CAD build for the part. Positions are in the model's coordinates, mm. Face numbers are marked on the shaded views. A direction names the side the tool comes from. Give positions to 0.01 mm unless a question says otherwise; leave off trailing zeros. Write each loop counter-clockwise with the first axis right and the second up, starting at its lowest first coordinate (ties: lowest second). Pieces come first, ordered by that corner, then holes. Notation, with made-up numbers: (63, 74) -> (118, 74) arc R24 cw to (118, 112) -> close; hole circle Ø4 at (1, -4). An arc over 180 degrees is marked (long way). Answer in a Markdown table with one row per item. Add a question column.
```python
from build123d import *

# Parameters (mm, degrees)
SKETCH1_R           = 1.8
SKETCH1_R_2         = 3.15
SKETCH1_R_3         = 8.05
SKETCH1_R_4         = 2.3
SKETCH1_R_5         = 19.05
SKETCH1_R_6         = 7.8
SKETCH1_R_7         = 1.3
SKETCH1_R_8         = 3.45
SKETCH1_W           = 98.2
SKETCH1_H           = 40.9
BOSS_EXTRUDE1_DEPTH = 3.2
BOSS_EXTRUDE2_START = 30
BOSS_EXTRUDE2_DEPTH = 30
FILLET1_R           = 4.8
SKETCH20_R          = 2.3
CUT_EXTRUDE8_DEPTH  = 10
SKETCH6_R           = 5
SKETCH6_R_2         = 2.3
BOSS_EXTRUDE3_DEPTH = 50
SKETCH12_W          = 192.98
SKETCH12_H          = 3.2
BOSS_EXTRUDE7_DEPTH = 15
SKETCH8_R           = 2.3
CUT_EXTRUDE2_DEPTH  = 10
SKETCH19_W          = 14
SKETCH19_H          = 60
CUT_EXTRUDE7_DEPTH  = 10
BOSS_EXTRUDE8_START = -30
SKETCH21_W          = 3.6
SKETCH21_H          = 22.135238484
SKETCH21_W_2        = 34.225238484
SKETCH21_H_2        = 3.6
BOSS_EXTRUDE8_DEPTH = 30
FILLET5_R           = 3
FILLET6_R           = 8


with BuildPart() as part:
    # Sketch1 → Boss-Extrude1 (new body)
    with BuildSketch(Plane(origin=(0, 0, 0), x_dir=(0, 0, -1), z_dir=(1, 0, 0))):
        with BuildLine():
            Line((-52.79, 54.2), (52.79, 54.2))
            ThreePointArc((52.79, 54.2), (91.185898218, 38.295898218), (107.09, -0.1))
            Line((107.09, -0.1), (107.09, -120.8))
            Line((107.09, -120.8), (-107.09, -120.8))
            Line((-107.09, -120.8), (-107.09, -0.1))
            ThreePointArc((-107.09, -0.1), (-91.185898218, 38.295898218), (-52.79, 54.2))
        make_face()
        with Locations((46.5, 27.4)):
            Circle(SKETCH1_R, mode=Mode.SUBTRACT)
        with Locations((-46.5, -27.6)):
            Circle(SKETCH1_R, mode=Mode.SUBTRACT)
        with Locations((-46.5, 27.4)):
            Circle(SKETCH1_R, mode=Mode.SUBTRACT)
        with Locations((46.5, -27.6)):
            Circle(SKETCH1_R, mode=Mode.SUBTRACT)
        with Locations((57.25, -0.1)):
            Circle(SKETCH1_R_2, mode=Mode.SUBTRACT)
        with Locations((68.55, -0.1)):
            Circle(SKETCH1_R_2, mode=Mode.SUBTRACT)
        with Locations((79.85, -0.1)):
            Circle(SKETCH1_R_2, mode=Mode.SUBTRACT)
        with Locations((91.15, -0.1)):
            Circle(SKETCH1_R_2, mode=Mode.SUBTRACT)
        with Locations((71.533650814, -45.1)):
            Circle(SKETCH1_R_3, mode=Mode.SUBTRACT)
        with Locations((87.09, -60.656349186)):
            Circle(SKETCH1_R_3, mode=Mode.SUBTRACT)
        with Locations((71.533650814, -76.212698372)):
            Circle(SKETCH1_R_3, mode=Mode.SUBTRACT)
        with Locations((55.977301628, -91.769047558)):
            Circle(SKETCH1_R_3, mode=Mode.SUBTRACT)
        with Locations((40.420952442, -107.325396744)):
            Circle(SKETCH1_R_3, mode=Mode.SUBTRACT)
        with Locations((55.977301628, -60.656349186)):
            Circle(SKETCH1_R_3, mode=Mode.SUBTRACT)
        with Locations((40.420952442, -76.212698372)):
            Circle(SKETCH1_R_3, mode=Mode.SUBTRACT)
        with Locations((24.864603256, -91.769047558)):
            Circle(SKETCH1_R_3, mode=Mode.SUBTRACT)
        with Locations((-87.45, -106.35)):
            Circle(SKETCH1_R_4, mode=Mode.SUBTRACT)
        with Locations((-52.45, -106.35)):
            Circle(SKETCH1_R_4, mode=Mode.SUBTRACT)
        with Locations((-52.45, -64.55)):
            Circle(SKETCH1_R_4, mode=Mode.SUBTRACT)
        with Locations((-87.45, -64.55)):
            Circle(SKETCH1_R_4, mode=Mode.SUBTRACT)
        with Locations((-69.1, -85.45)):
            Circle(SKETCH1_R_5, mode=Mode.SUBTRACT)
        with Locations((-81.9, -25.1)):
            Circle(SKETCH1_R_6, mode=Mode.SUBTRACT)
        with Locations((46.42, 37.2)):
            Circle(SKETCH1_R, mode=Mode.SUBTRACT)
        with Locations((0, 37.2)):
            Circle(SKETCH1_R, mode=Mode.SUBTRACT)
        with Locations((23.21, 34.55)):
            Circle(SKETCH1_R, mode=Mode.SUBTRACT)
        with Locations((23.21, -35.45)):
            Circle(SKETCH1_R, mode=Mode.SUBTRACT)
        with Locations((-29.2, -38.8)):
            Circle(SKETCH1_R_7, mode=Mode.SUBTRACT)
        with Locations((-13, -38.8)):
            Circle(SKETCH1_R_7, mode=Mode.SUBTRACT)
        with Locations((-13, -114.8)):
            Circle(SKETCH1_R_7, mode=Mode.SUBTRACT)
        with Locations((-29.2, -114.8)):
            Circle(SKETCH1_R_7, mode=Mode.SUBTRACT)
        with Locations((91.15, -12.7)):
            Circle(SKETCH1_R_8, mode=Mode.SUBTRACT)
        with Locations((79.85, -12.7)):
            Circle(SKETCH1_R_8, mode=Mode.SUBTRACT)
        with Locations((68.55, -12.7)):
            Circle(SKETCH1_R_8, mode=Mode.SUBTRACT)
        with Locations((57.25, -12.7)):
            Circle(SKETCH1_R_8, mode=Mode.SUBTRACT)
        Rectangle(SKETCH1_W, SKETCH1_H, mode=Mode.SUBTRACT)
    extrude(amount=BOSS_EXTRUDE1_DEPTH)

    # Sketch3 → Boss-Extrude2 (add)
    with BuildSketch(Plane.ZY.offset(BOSS_EXTRUDE2_START)):
        with BuildLine():
            Line((-107.09, -0.1), (-107.09, -120.8))
            Line((-107.09, -120.8), (107.09, -120.8))
            Line((107.09, -120.8), (107.09, -0.1))
            ThreePointArc((107.09, -0.1), (91.185898218, 38.295898218), (52.79, 54.2))
            Line((52.79, 54.2), (-52.79, 54.2))
            ThreePointArc((-52.79, 54.2), (-91.185898218, 38.295898218), (-107.09, -0.1))
        make_face()
        with BuildLine():
            Line((-103.89, -0.1), (-103.89, -117.6))
            Line((-103.89, -117.6), (103.89, -117.6))
            Line((103.89, -117.6), (103.89, -0.1))
            ThreePointArc((103.89, -0.1), (88.923156519, 36.033156519), (52.79, 51))
            Line((52.79, 51), (-52.79, 51))
            ThreePointArc((-52.79, 51), (-88.923156519, 36.033156519), (-103.89, -0.1))
        make_face(mode=Mode.SUBTRACT)
    extrude(amount=-BOSS_EXTRUDE2_DEPTH)

    # Fillet1
    fillet1_edges = [part.edges().sort_by_distance(p)[0] for p in [
        (0, 36.033156519, -88.923156519),
        (0, -58.85, -103.89),
        (0, -58.85, 103.89),
        (0, 36.033156519, 88.923156519),
        (0, 51, 0),
    ]]
    fillet(fillet1_edges, radius=FILLET1_R)

    # Sketch20 → Cut-Extrude8 (cut)
    with BuildSketch(Plane(origin=(3.2, 0, 0), x_dir=(0, 0, -1), z_dir=(1, 0, 0))):
        with Locations((-65, 9.2)):
            Circle(SKETCH20_R)
        with Locations((0, -51.8)):
            Circle(SKETCH20_R)
        with Locations((-50, -45.8)):
            Circle(SKETCH20_R)
        with Locations((65, 24.2)):
            Circle(SKETCH20_R)
        with Locations((80, -100.8)):
            Circle(SKETCH20_R)
    extrude(amount=-CUT_EXTRUDE8_DEPTH, mode=Mode.SUBTRACT)

    # Sketch6 → Boss-Extrude3 (add)
    # profile 1 of 5: a face of its own
    with BuildSketch(Plane.ZY):
        with Locations((65, 9.2)):
            Circle(SKETCH6_R)
        with Locations(Location((65, 9.2, 0), (0, 0, 180))):
            Circle(SKETCH6_R_2, mode=Mode.SUBTRACT)
    # profile 2 of 5: a face of its own
    with BuildSketch(Plane.ZY):
        with Locations((-65, 24.2)):
            Circle(SKETCH6_R)
        with Locations(Location((-65, 24.2, 0), (0, 0, 180))):
            Circle(SKETCH6_R_2, mode=Mode.SUBTRACT)
    # profile 3 of 5: a face of its own
    with BuildSketch(Plane.ZY):
        with Locations((-80, -100.8)):
            Circle(SKETCH6_R)
        with Locations(Location((-80, -100.8, 0), (0, 0, 180))):
            Circle(SKETCH6_R_2, mode=Mode.SUBTRACT)
    # profile 4 of 5: a face of its own
    with BuildSketch(Plane.ZY):
        with Locations((50, -45.8)):
            Circle(SKETCH6_R)
        with Locations(Location((50, -45.8, 0), (0, 0, 180))):
            Circle(SKETCH6_R_2, mode=Mode.SUBTRACT)
    # profile 5 of 5: a face of its own
    with BuildSketch(Plane.ZY):
        with Locations((0, -51.8)):
            Circle(SKETCH6_R)
        with Locations(Location((0, -51.8, 0), (0, 0, 180))):
            Circle(SKETCH6_R_2, mode=Mode.SUBTRACT)
    extrude(amount=BOSS_EXTRUDE3_DEPTH)

    # Sketch12 → Boss-Extrude7 (add)
    with BuildSketch(Plane.ZY.offset(30)):
        with Locations((0, -119.2)):
            Rectangle(SKETCH12_W, SKETCH12_H)
    extrude(amount=BOSS_EXTRUDE7_DEPTH)

    # Sketch8 → Cut-Extrude2 (cut)
    with BuildSketch(Plane.XZ.offset(120.8)):
        with Locations(Location((-14.6, 92.09, 0), (0, 0, 270))):
            Circle(SKETCH8_R)
        with Locations(Location((-34.6, 92.09, 0), (0, 0, 270))):
            Circle(SKETCH8_R)
        with Locations(Location((-14.6, -92.09, 0), (0, 0, 270))):
            Circle(SKETCH8_R)
        with Locations(Location((-34.6, -92.09, 0), (0, 0, 270))):
            Circle(SKETCH8_R)
    extrude(amount=-CUT_EXTRUDE2_DEPTH, mode=Mode.SUBTRACT)

    # Sketch19 → Cut-Extrude7 (cut)
    with BuildSketch(Plane(origin=(0, 54.2, 0), x_dir=(1, 0, 0), z_dir=(0, 1, 0))):
        with Locations((-23, 22.79)):
            Rectangle(SKETCH19_W, SKETCH19_H)
    extrude(amount=-CUT_EXTRUDE7_DEPTH, mode=Mode.SUBTRACT)

    # Sketch21 → Boss-Extrude8 (add)
    with BuildSketch(Plane(origin=(0, 0, 0), x_dir=(0, 0, -1), z_dir=(1, 0, 0)).offset(BOSS_EXTRUDE8_START)):
        with BuildLine():
            Line((103.89, -102.6), (85, -102.6))
            Line((85, -102.6), (84.664761516, -102.6))
            ThreePointArc((84.664761516, -102.6), (85, -100.8), (84.664761516, -99))
            Line((84.664761516, -99), (85, -99))
            Line((85, -99), (103.89, -99))
            Line((103.89, -99), (103.89, -102.6))
        make_face()
        with Locations((65, 39.932380758)):
            Rectangle(SKETCH21_W, SKETCH21_H)
        with Locations((-86.777380758, 9.2)):
            Rectangle(SKETCH21_W_2, SKETCH21_H_2)
    extrude(amount=BOSS_EXTRUDE8_DEPTH)

    # Fillet5
    fillet5_edges = [part.edges().sort_by_distance(p)[0] for p in [
        (0, -105.715475947, -79.084524053),
        (0, -99, -91.877380758),
        (0, -102.6, -91.877380758),
        (-17.4, -102.6, -103.89),
        (-15, -99, -84.664761516),
        (-1.40588745, -102.6, -102.48411255),
        (-17.4, -99, -103.89),
        (-1.40588745, -99, -102.48411255),
        (-15, -102.6, -84.664761516),
    ]]
    fillet(fillet5_edges, radius=FILLET5_R)

    # Fillet6
    fillet6_edges = [part.edges().sort_by_distance(p)[0] for p in [
        (3.2, 38.295898218, 91.185898218),
        (3.2, -60.45, 107.09),
        (3.2, -60.45, -107.09),
        (3.2, 38.295898218, -91.185898218),
        (3.2, 54.2, 0),
    ]]
    fillet(fillet6_edges, radius=FILLET6_R)


solid = part.part
```
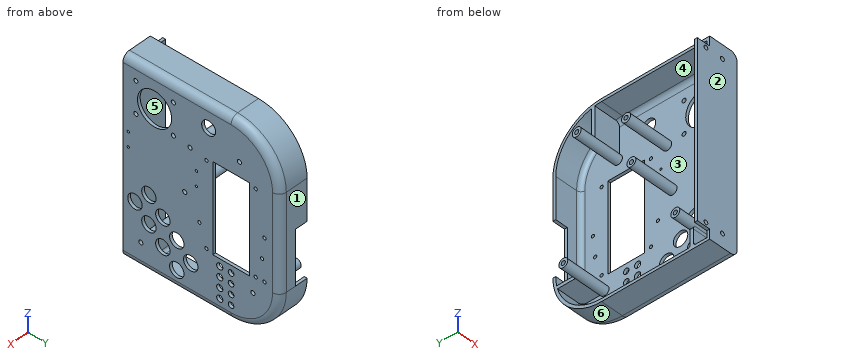
Item 1: Which spindle directions (+Z, -Z, +X, -X, +Y, -Y) get a long thin tool onto all of the face, cutting with end or side? Do the marked faces 5 and 6. Say none if no direction does.
Item 2: Slice it at B-B, the plane y = -81. List the corners of the cut face in (x, z).
Item 3: Mould opens along Y. For the marked faces 1, 2, 3 and 4 say: released by +Y, released by -Y, zero draft, split by the parting line, or undercut.
Item 4: Probe L1, parallel to Z at x = -25, y = -21.5; L2, parallel to Y at x = -19, z = -91.5; L3, parallel to Y at x = -4.5, z = 96.5. List the from-to ranges inside material, lowest first. Write a range as from..to.
Item 5: Drop flat-ended pins along their axis: pin 1 Ø21 at (y, z) = (-107.33, -40.42) entering from +X; pin 2 Ø10 at (x, y) = (-40.5, 20) entering from -Z; pin 3 Ø9 at (x, z) = (-15.5, 94.5) entering from +Y; pin 4 Ø3.5 at (y, z) = (-38.8, 13) entering from -X. Give the stop position or say it passes through.
Item 6: Slice it at A-A, the plane x = -34.6. State how many separate pieces and enclosed holes the cut face has, then the cut area to 3 significant figures.
Answer key:
| question | item | result |
|---|---|---|
| 1 | face 5 | -X |
| 1 | face 6 | -Z, +X, -X, +Y |
| 2 | outline | (-30, -107.09) -> (-4.8, -107.09) arc R8 ccw to (3.2, -99.09) -> (3.2, -78.01) -> (0, -78.01) -> (0, -99.09) arc R4.8 cw to (-4.8, -103.89) -> (-30, -103.89) -> close; (-30, 103.89) -> (-4.8, 103.89) arc R4.8 cw to (0, 99.09) -> (0, 87.62) -> (3.2, 87.62) -> (3.2, 99.09) arc R8 ccw to (-4.8, 107.09) -> (-30, 107.09) -> close; (0, -65.06) -> (3.2, -65.06) -> (3.2, -46.89) -> (0, -46.89) -> close; (0, -33.95) -> (3.2, -33.95) -> (3.2, 50.58) -> (0, 50.58) -> close |
| 3 | face 1 | released by +Y |
| 3 | face 2 | released by -Y |
| 3 | face 3 | undercut |
| 3 | face 4 | undercut |
| 4 | L1 | z = -107.09..-103.89, 103.89..107.09 |
| 4 | L2 | y = -120.8..-117.6, -102.6..-99, 33.26..37.98 |
| 4 | L3 | y = -120.8..-117.6, 7.4..11, 26.35..32.11 |
| 5 | pin 1 | stops at x = 3.2 |
| 5 | pin 2 | stops at z = -70 |
| 5 | pin 3 | stops at y = 39.45 |
| 5 | pin 4 | stops at x = 0 |
| 6 | separate pieces | 8 |
| 6 | enclosed holes | 5 |
| 6 | area | 898 mm² |
